Here's how the part is built. I have some questions about the finished solid (model axes, mm). A direction names the side the tool comes from. Coordinates: 2 decimals unless noted, no trailing zeros. Order: outer loops, then holes, each group sorted by start corner. A loop starts at its lowest first (then second) coordinate and runs counter-clockwise, first axis right, second up.
```python
from build123d import *

# Parameters (mm, degrees)
BOSS_EXTRUDE1_DEPTH = 5
SKETCH2_R           = 21
BOSS_EXTRUDE3_DEPTH = 7.5
SKETCH3_R           = 12
BOSS_EXTRUDE4_DEPTH = 7.5
SKETCH4_R           = 21
BOSS_EXTRUDE6_DEPTH = 7.5
SKETCH5_R           = 12
BOSS_EXTRUDE7_DEPTH = 7.5
SKETCH6_R           = 11
CUT_EXTRUDE1_DEPTH  = 69
SKETCH7_R           = 6
CUT_EXTRUDE2_DEPTH  = 69
CUT_EXTRUDE4_DEPTH  = 2
CUT_EXTRUDE5_DEPTH  = 2


with BuildPart() as part:
    # Sketch1 → Boss-Extrude1 (new, symmetric)
    with BuildSketch(Plane(origin=(0, 0, 0), x_dir=(1, 0, 0), z_dir=(0, 1, 0))):
        Polygon((90, -12), (0, -21), (0, 21), (90, 12), align=None)
    extrude(amount=BOSS_EXTRUDE1_DEPTH, both=True)

    # Sketch2 → Boss-Extrude3 (add, symmetric)
    with BuildSketch(Plane(origin=(0, 5, 0), x_dir=(1, 0, 0), z_dir=(0, 1, 0))):
        with Locations(Location((0, 0, 0), (0, 0, 270))):
            Circle(SKETCH2_R)
    extrude(amount=BOSS_EXTRUDE3_DEPTH, both=True)

    # Sketch3 → Boss-Extrude4 (add, symmetric)
    with BuildSketch(Plane(origin=(0, 5, 0), x_dir=(1, 0, 0), z_dir=(0, 1, 0))):
        with Locations(Location((90, 0, 0), (0, 0, 270))):
            Circle(SKETCH3_R)
    extrude(amount=BOSS_EXTRUDE4_DEPTH, both=True)

    # Sketch4 → Boss-Extrude6 (add, symmetric)
    with BuildSketch(Plane.XZ.offset(5)):
        with Locations(Location((0, 0, 0), (0, 0, 270))):
            Circle(SKETCH4_R)
    extrude(amount=BOSS_EXTRUDE6_DEPTH, both=True)

    # Sketch5 → Boss-Extrude7 (add, symmetric)
    with BuildSketch(Plane.XZ.offset(5)):
        with Locations(Location((90, 0, 0), (0, 0, 270))):
            Circle(SKETCH5_R)
    extrude(amount=BOSS_EXTRUDE7_DEPTH, both=True)

    # Sketch6 → Cut-Extrude1 (cut)
    with BuildSketch(Plane(origin=(0, 12.5, 0), x_dir=(1, 0, 0), z_dir=(0, 1, 0))):
        with Locations(Location((0, 0, 0), (0, 0, 270))):
            Circle(SKETCH6_R)
    extrude(amount=-CUT_EXTRUDE1_DEPTH, mode=Mode.SUBTRACT)

    # Sketch7 → Cut-Extrude2 (cut)
    with BuildSketch(Plane(origin=(0, 12.5, 0), x_dir=(1, 0, 0), z_dir=(0, 1, 0))):
        with Locations(Location((90, 0, 0), (0, 0, 270))):
            Circle(SKETCH7_R)
    extrude(amount=-CUT_EXTRUDE2_DEPTH, mode=Mode.SUBTRACT)

    # Sketch8 → Cut-Extrude4 (cut)
    with BuildSketch(Plane(origin=(0, 5, 0), x_dir=(1, 0, 0), z_dir=(0, 1, 0))):
        with BuildLine():
            Line((24.562692553, 12.477391073), (73.943240769, 7.677349154))
            ThreePointArc((73.943240769, 7.677349154), (75.435017265, 6.76369448), (75.637490363, 5.026119554))
            ThreePointArc((75.637490363, 5.026119554), (74.783444514, 0), (75.637490363, -5.026119554))
            ThreePointArc((75.637490363, -5.026119554), (75.435017265, -6.76369448), (73.943240769, -7.677349154))
            Line((73.943240769, -7.677349154), (24.562692553, -12.477391073))
            ThreePointArc((24.562692553, -12.477391073), (21.879607854, -11.300975456), (21.478465069, -8.398910386))
            ThreePointArc((21.478465069, -8.398910386), (23.062223601, 0), (21.478465069, 8.398910386))
            ThreePointArc((21.478465069, 8.398910386), (21.879607854, 11.300975456), (24.562692553, 12.477391073))
        make_face()
    extrude(amount=-CUT_EXTRUDE4_DEPTH, mode=Mode.SUBTRACT)

    # Sketch9 → Cut-Extrude5 (cut)
    with BuildSketch(Plane.XZ.offset(5)):
        with BuildLine():
            Line((75.653851905, 8.117723123), (25.352219693, 12.951931944))
            ThreePointArc((25.352219693, 12.951931944), (22.666288444, 11.767102867), (22.27748823, 8.857312323))
            ThreePointArc((22.27748823, 8.857312323), (23.973703582, 0), (22.27748823, -8.857312323))
            ThreePointArc((22.27748823, -8.857312323), (22.666288444, -11.767102867), (25.352219693, -12.951931944))
            Line((25.352219693, -12.951931944), (75.653851905, -8.117723123))
            ThreePointArc((75.653851905, -8.117723123), (77.179932686, -7.151839338), (77.305529846, -5.35015141))
            ThreePointArc((77.305529846, -5.35015141), (76.224162726, 0), (77.305529846, 5.35015141))
            ThreePointArc((77.305529846, 5.35015141), (77.179932686, 7.151839338), (75.653851905, 8.117723123))
        make_face()
    extrude(amount=-CUT_EXTRUDE5_DEPTH, mode=Mode.SUBTRACT)


solid = part.part
```
Q1. If we section it at A-A on z = 0: Write out the boundary of the cut face in (x, y).
Q2. If we section it at D-D on z = 16: Write out the boundary of the cut face in (x, y).
Q3. I need wall thicknesses on L1, parallel to X at y = 7, z = 0; L2, parallel to X at y = -4.5, z = 0; L3, parallel to X at y = 0.75, z = 0. Which ranges of each line are inside material? Lowest first, please.
Q4. If we section it at C-C on y = 9.5: Write out the boundary of the cut face in (x, z), then the cut area to 3 significant figures.
Q5. If we section it at B-B on x = 0: Write out the boundary of the cut face in (y, z).
Q6. We'd pull the mould along Z, two halves only. Please class faces 6 (the flat face through (50.15, -4.01, -10.57)), 7 (the flat face through (46.48, 0.07, -16.35)), 8 (the flat face through (47.68, 0.07, 16.23)), 9 (the cylindrical face through (22.69, -4.01, 11.8)): pulls with the +Z half, pulls with the -Z half, needs draft (parallel to the pull), parting line crosses it, or undercut.
Q7. For faces 1 (the cylindrical face through (21.854, 4.014, -11.267)), 2 (the flat face through (50.86, -4.01, 10.5)), 3 (the flat face through (-9, -12.5, -9)), 4 (the cylindrical face through (20.954, 5.731, 1.384)), 5 (the flat face through (88, 12.5, -6)), which set-ups out of +Z, -Z, +X, -X, +Y, -Y let a thin tool reach every point of the face, with its end or its side?
Q8. Will these pins go through, and if not, where does the flat tip stop? pin 1 (12 mm diameter, centred on x = 87, y = -8.5, fed in from -Z); pin 2 (20.5 mm diameter, centred on x = 36.5, z = -5.5, fed in from -Y); pin 3 (12.5 mm diameter, centred on x = 59.5, z = -1.5, fed in from +Y); pin 4 (13 mm diameter, centred on x = 0, z = 0, fed in from -Y).
Reply:
1. outline: (-21, -12.5) - (-11, -12.5) - (-11, 12.5) - (-21, 12.5) - close; (11, -12.5) - (21, -12.5) - (21, -5) - (23.97, -5) - (23.97, -3) - (76.22, -3) - (76.22, -5) - (78, -5) - (78, -12.5) - (84, -12.5) - (84, 12.5) - (78, 12.5) - (78, 5) - (74.78, 5) - (74.78, 3) - (23.06, 3) - (23.06, 5) - (21, 5) - (21, 12.5) - (11, 12.5) - close; (96, -12.5) - (102, -12.5) - (102, 12.5) - (96, 12.5) - close
2. outline: (-13.6, -12.5) - (13.6, -12.5) - (13.6, -5) - (50, -5) - (50, 5) - (13.6, 5) - (13.6, 12.5) - (-13.6, 12.5) - close
3. L1: x = -21 to -11, 11 to 21, 78 to 84, 96 to 102
3. L2: x = -21 to -11, 11 to 23.97, 76.22 to 84, 96 to 102
3. L3: x = -21 to -11, 11 to 84, 96 to 102
4. outline: circle Ø42 at (0, 0); circle Ø24 at (90, 0); hole circle Ø22 at (0, 0); hole circle Ø12 at (90, 0)
4. area: 1,340 mm2
5. outline: (-12.5, -21) - (12.5, -21) - (12.5, -11) - (-12.5, -11) - close; (-12.5, 11) - (12.5, 11) - (12.5, 21) - (-12.5, 21) - close
6. face 6: undercut
6. face 7: pulls with the -Z half
6. face 8: pulls with the +Z half
6. face 9: undercut
7. face 1: +Y
7. face 2: -Y
7. face 3: +Z, -Z, +X, -X, -Y
7. face 4: none
7. face 5: +Z, -Z, +X, -X, +Y
8. pin 1: stops at z = -12.79
8. pin 2: stops at y = -5
8. pin 3: stops at y = 3
8. pin 4: passes through
